from build123d import *

# Parameters (mm, degrees)
BOSS_EXTRUDE1_DEPTH = 3
FILLET1_R           = 2.54


with BuildPart() as part:
    # Sketch1 → Boss-Extrude1 (new, symmetric)
    with BuildSketch(Plane.XY):
        Polygon((-120.825, -28.575), (-120.825, 28.575), (-101.775, 28.575), (-89.075, -3.175), (89.075, -3.175), (101.775, 28.575), (120.825, 28.575), (120.825, -28.575), align=None)
        with BuildLine():
            Line((-112.975, 22.225), (-112.975, -22.225))
            ThreePointArc((-112.975, -22.225), (-114.475, -23.725), (-115.975, -22.225))
            Line((-115.975, -22.225), (-115.975, 22.225))
            ThreePointArc((-115.975, 22.225), (-114.475, 23.725), (-112.975, 22.225))
        make_face(mode=Mode.SUBTRACT)
        with BuildLine():
            Line((115.975, 22.225), (115.975, -22.225))
            ThreePointArc((115.975, -22.225), (114.475, -23.725), (112.975, -22.225))
            Line((112.975, -22.225), (112.975, 22.225))
            ThreePointArc((112.975, 22.225), (114.475, 23.725), (115.975, 22.225))
        make_face(mode=Mode.SUBTRACT)
    extrude(amount=BOSS_EXTRUDE1_DEPTH, both=True)

    # Fillet1
    fillet1_edges = [part.edges().sort_by_distance(p)[0] for p in [
        (120.825, 28.575, 0),
        (120.825, -28.575, 0),
        (-120.825, -28.575, 0),
        (-120.825, 28.575, 0),
        (-101.775, 28.575, 0),
        (-89.075, -3.175, 0),
        (89.075, -3.175, 0),
        (101.775, 28.575, 0),
    ]]
    fillet(fillet1_edges, radius=FILLET1_R)


solid = part.part
Build history of the part. All positions in model axes, mm. A direction names the side the tool comes from. Round coordinates to 2 decimals unless told otherwise and drop trailing zeros. Write each loop counter-clockwise with the first axis right and the second up, starting at its lowest first coordinate (ties: lowest second). Pieces come first, ordered by that corner, then holes. Notation, with made-up numbers: M -12.5,88 L 33.5,88 A28 ccw 33.5,107 Z; hole C -31,37.25 d10. An arc over 180 degrees is marked long. Answer as a JSON object with one key per item and string values. Group by question number.
(1) Cut at B-B (z = -1.7). Give the cut face in (x, y) (3 decimals).
(2) Cut at A-A (y = -13). Give the cut face in (x, z) (3 decimals).
(3) Cut at D-D (x = -24). Give the cut face in (y, z) (3 decimals).
(4) Mould opens along X. For faces 1 (the flat face through (2, -28.575, 0)), 2 (the flat face through (-112.975, 0, 0)), 3 (the flat face through (120.825, 0, 0)) say: pulls with the +X half, pulls with the -X half, needs draft (parallel to the pull), parting line crosses it, or undercut.
(5) Flat gauge pin, fed straight in: pin 1 (2 mm diameter, centred on x = -21.5, z = -2, fed in from +Y) (3 decimals). Where does the tip first touch, or does it go through?
(6) Which spindle directions (+Z, -Z, +X, -X, +Y, -Y) get a long thin tool onto all of the face, cutting with end or side? Do faces 4 (the flat face through (-1, -3.175, 0)), 5 (the flat face through (-111, 28.575, 0)), 6 (the flat face through (112.975, 0, 0)). Say none if no direction does.
(7) Cut at C-C (y = 6). Give the cut face in (x, z) (3 decimals).
(8) Drill centre lines: L1, parallel to X at y = -18.5, z = -2 (3 decimals); L2, parallel to X at y = 23.5, z = 0 (3 decimals); L3, parallel to X at y = 19, z = -1.3 (3 decimals). Where is each one in solid material? Low to high.
Responses:
{
 "1": {"outline": "M -120.825,-26.035 A2.54 ccw -118.285,-28.575 L 118.285,-28.575 A2.54 ccw 120.825,-26.035 L 120.825,26.035 A2.54 ccw 118.285,28.575 L 103.495,28.575 A2.54 ccw 101.136,26.978 L 89.714,-1.578 A2.54 cw 87.355,-3.175 L -87.355,-3.175 A2.54 cw -89.714,-1.578 L -101.136,26.978 A2.54 ccw -103.495,28.575 L -118.285,28.575 A2.54 ccw -120.825,26.035 Z; hole M -115.975,-22.225 A1.5 ccw -112.975,-22.225 L -112.975,22.225 A1.5 ccw -115.975,22.225 Z; hole M 112.975,-22.225 A1.5 ccw 115.975,-22.225 L 115.975,22.225 A1.5 ccw 112.975,22.225 Z"},
 "2": {"outline": "M -120.825,-3 L -115.975,-3 L -115.975,3 L -120.825,3 Z; M -112.975,-3 L 112.975,-3 L 112.975,3 L -112.975,3 Z; M 115.975,-3 L 120.825,-3 L 120.825,3 L 115.975,3 Z"},
 "3": {"outline": "M -28.575,-3 L -3.175,-3 L -3.175,3 L -28.575,3 Z"},
 "4": {"face 1": "needs draft", "face 2": "undercut", "face 3": "pulls with the +X half"},
 "5": {"pin 1": "stops at y = -3.175"},
 "6": {"face 4": "+Z, -Z, +Y", "face 5": "+Z, -Z, +X, -X, +Y", "face 6": "+Z, -Z"},
 "7": {"outline": "M -120.825,-3 L -115.975,-3 L -115.975,3 L -120.825,3 Z; M -112.975,-3 L -92.745,-3 L -92.745,3 L -112.975,3 Z; M 92.745,-3 L 112.975,-3 L 112.975,3 L 92.745,3 Z; M 115.975,-3 L 120.825,-3 L 120.825,3 L 115.975,3 Z"},
 "8": {"L1": "x = -120.825 to -115.975, -112.975 to 112.975, 115.975 to 120.825", "L2": "x = -120.825 to -115.265, -113.685 to -99.745, 99.745 to 113.685, 115.265 to 120.825", "L3": "x = -120.825 to -115.975, -112.975 to -97.945, 97.945 to 112.975, 115.975 to 120.825"}
}
